Source: CAD feature listing. Evaluate the final solid. Frame: model axes, mm. A direction names the side the tool comes from. Give positions to 0.01 mm unless a question says otherwise; leave off trailing zeros. Loops run counter-clockwise (first coordinate to the right, second up) from the corner with the lowest first, then second, coordinate; pieces in that order, holes last. Notation, with made-up numbers: M 15.25,69 L 39.25,69 A19 cw 39.25,90 Z; hole C 76,86.5 d11. An arc over 180 degrees is marked long. Answer in a Markdown table with one row per item.
Autodesk Inventor part; units mm, degrees
ref_plane "YZ Plane" through (0, 0, 0) normal (1, 0, 0) x (0, 1, 0)
ref_plane "XZ Plane" through (0, 0, 0) normal (0, 1, 0) x (-1, 0, 0)
ref_plane "XY Plane" through (0, 0, 0) normal (0, 0, 1) x (1, 0, 0)
sketch "Эскиз1" plane through (0, 0, 0) normal (0, 0, 1) x (1, 0, 0)
  line L0 (0, 0) -> (0, 8)
  line L1 (0, 8) -> (0, 16)
  line L2 (0, 16) -> (69, 16)
  line L3 (69, 16) -> (69, 0)
  line L4 (69, 0) -> (49, 0)
  line L5 (49, 0) -> (49, 8)
  line L6 (49, 8) -> (32, 8)
  line L7 (32, 8) -> (32, 16)
  line L8 (0, 16) -> (49, 16)
  line L9 (49, 16) -> (49, 17)
  circle A0 centre (49, 17) radius 3
  point P0 (51.8284, 16)
  point P1 (46.1716, 16)
  dimension "d0" = 8
  dimension "d1" = 8
  dimension "d2" = 69
  dimension "d3" = 20
  dimension "d4" = 17
  dimension "d6" = 32
  dimension "d7" = 49
  dimension "d8" = 49
  dimension "d9" = 1
  dimension "d10" = 6
revolve "Вращение1" add sketch "Эскиз1" angle 360 about axis through (0, 8, 0) along (0, 1, 0) contours L2 A0 L3 L4 L5 L6 L7
sketch "Эскиз2" plane through (0, 16, 0) normal (0, 1, 0) x (1, 0, 0)
  line L0 (0, 0) -> (38.5673, 45.9627)
  line L1 (0, 0) -> (60, 0) construction
  line L2 (0, 0) -> (-30, 51.9615)
  line L3 (0, 0) -> (60, 0) construction
  line L4 (0, 0) -> (-10.4189, -59.0885)
  line L5 (0, 0) -> (60, 0) construction
  circle A0 centre (-30, 51.9615) radius 3
  circle A1 centre (38.5673, 45.9627) radius 3
  circle A2 centre (-10.4189, -59.0885) radius 3
  dimension "d11" = 60
  dimension "d12" = 50
  dimension "d13" = 60
  dimension "d14" = 120
  dimension "d15" = 60
  dimension "d16" = 100
  dimension "d17" = 6
  dimension "d18" = 6
  dimension "d19" = 6
extrude "Выдавливание1" cut sketch "Эскиз2" against normal through all
properties part number "Корпус дросселя_CPY" material "Чугун, серый"
Q1. Contact query for flat-ended pins moving along their axis: pin 1 Ø3 at (y, z) = (11, -34.5) entering from +X; pin 2 Ø5 at (x, y) = (33, 10) entering from +Z; pin 3 Ø2 at (y, z) = (8, -45) entering from +X. Output: stop coordinate, or through.
Values follow:
| item | result |
|---|---|
| pin 1 | x = 60.6 |
| pin 2 | z = 61.89 |
| pin 3 | x = 53.15 |
Q2. Section query C-C (y = 4.75). Output: boundary loops of the cut face in (x, z), plus the area to 3 significant figures.
Values follow:
| item | result |
|---|---|
| outline | C 0,0 d138; hole C 0,0 d98; hole C -30,-51.96 d6; hole C -10.42,59.09 d6; hole C 38.57,-45.96 d6 |
| area | 7,330 mm^2 |
Q3. Section query B-B (z = 0). Output: boundary loops of the cut face in (x, y), plus the area to 4 significant figures.
Values follow:
| item | result |
|---|---|
| outline | M -69,0 L -49,0 L -49,8 L -32,8 L -32,16 L -46.17,16 A3 cw -51.83,16 L -69,16 Z; M 32,8 L 49,8 L 49,0 L 69,0 L 69,16 L 51.83,16 A3 cw 46.17,16 L 32,16 Z |
| area | 895.5 mm^2 |
Q4. Section query D-D (x = -30). Give the number of separate pieces and of enclosed holes in the cut face, plus the area to 3 significant figures.
Values follow:
| item | result |
|---|---|
| separate pieces | 3 |
| enclosed holes | 0 |
| area | 1,070 mm^2 |
Q5. Section query A-A (x = 0). Output: boundary loops of the cut face in (y, z).
Values follow:
| item | result |
|---|---|
| outline | M 0,-69 L 16,-69 L 16,-51.83 A3 cw 16,-46.17 L 16,-32 L 8,-32 L 8,-49 L 0,-49 Z; M 0,49 L 8,49 L 8,32 L 16,32 L 16,46.17 A3 cw 16,51.83 L 16,69 L 0,69 Z |
Q6. Mould query, pull axis Z, two halves, no side actions, for faces 1 (the cylindrical face through (-6.94, 12.06, 31.24)), 2 (the flat face through (-47, 0, 14.4)), 3 (the cylindrical face through (65.814, 7.888, 20.726)). Classes: +Z half, -Z half, draft (parallel to the pull), parting line (faces both ways), or undercut.
Values follow:
| item | result |
|---|---|
| face 1 | undercut |
| face 2 | draft |
| face 3 | parting line |
Q7. Ray query, probe 1 along X at (y, z) = (11.75, 0); probe 2 along Z at (x, y) = (0, 2.75); probe 3 along Z at (x, y) = (0, 14.75). Return the intervals inside material, ascending. Write a range as from..to.
Values follow:
| item | result |
|---|---|
| probe 1 | -69..-32, 32..69 |
| probe 2 | -69..-49, 49..69 |
| probe 3 | -69..-50.98, -47.02..-32, 32..47.02, 50.98..69 |
Q8. Reachability of faces 4 (the flat face through (10, 16, -31)), 5 (the flat face through (32, 8, 10)) from +Z, -Z, +X, -X, +Y, -Y: full face, straight path, thin tool, end or side. Return the list, or none.
Values follow:
| item | result |
|---|---|
| face 4 | +Z, -Z, +X, -X, +Y |
| face 5 | -Y |
